```python
from build123d import *

# Parameters (mm, degrees)
SKETCH2_W           = 30
SKETCH2_H           = 10
BOSS_EXTRUDE1_DEPTH = 6.35
SKETCH3_W           = 35.56
SKETCH3_H           = 10
CUT_EXTRUDE1_DEPTH  = 6.35


with BuildPart() as part:
    # Sketch2 → Boss-Extrude1 (new body)
    with BuildSketch(Plane.XY):
        Polygon((12.244662888, 165.1), (24.944662888, 165.1), (24.944662888, 158.75), (35.263412888, 158.75), (35.263412888, 150.8125), (32.882162888, 150.8125), (32.882162888, 147.6375), (35.263412888, 147.6375), (35.263412888, 144.4625), (40.025912888, 144.4625), (40.025912888, 147.6375), (42.407162888, 147.6375), (42.407162888, 150.8125), (40.025912888, 150.8125), (40.025912888, 158.75), (50.344662888, 158.75), (50.344662888, 165.1), (63.044662888, 165.1), (63.044662888, 158.75), (75.744662888, 158.75), (75.744662888, 6.35), (63.044662888, 6.35), (63.044662888, 0), (50.344662888, 0), (50.344662888, 6.35), (40.025912888, 6.35), (40.025912888, 14.2875), (42.407162888, 14.2875), (42.407162888, 17.4625), (40.025912888, 17.4625), (40.025912888, 20.6375), (35.263412888, 20.6375), (35.263412888, 17.4625), (32.882162888, 17.4625), (32.882162888, 14.2875), (35.263412888, 14.2875), (35.263412888, 6.35), (24.944662888, 6.35), (24.944662888, 0), (12.244662888, 0), (12.244662888, 6.35), (-0.455337112, 6.35), (-0.455337112, 158.75), (12.244662888, 158.75), align=None)
        with Locations((37.644662886, 55.8)):
            Rectangle(SKETCH2_W, SKETCH2_H, mode=Mode.SUBTRACT)
    extrude(amount=BOSS_EXTRUDE1_DEPTH)

    # Sketch3 → Cut-Extrude1 (cut)
    with BuildSketch(Plane.XY.offset(6.35)):
        with Locations((37.623375509, 55.8)):
            Rectangle(SKETCH3_W, SKETCH3_H)
    extrude(amount=-CUT_EXTRUDE1_DEPTH, mode=Mode.SUBTRACT)


solid = part.part
```
Read the model definition and answer for the solid it produces. Units are mm, in the model's axes. A direction names the side the tool comes from. Give positions to 0.01 mm unless a question says otherwise; leave off trailing zeros. Loops run counter-clockwise (first coordinate to the right, second up) from the corner with the lowest first, then second, coordinate; pieces in that order, holes last.
Item 1: The mould has two halves that part along Y. Classify faces 5 (the flat face through (19, 0, 3)), 6 (the flat face through (45, 158.75, 3)), 7 (the flat face through (37, 60.8, 3)): released by +Y, released by -Y, zero draft, split by the parting line, or undercut.
Item 2: Find the intervals of material crossed by line 1 along X through (y, z) = (153, 5.25); line 2 along X through (y, z) = (59, 6); line 3 along Y through (x, z) = (38, 0.5), in increasing order.
Item 3: The part is cut by section B-B (y = 146). Write down the section's boundary in (x, z), and give its area (3 significant figures).
Item 4: Each of these flat-tipped pins is pushed along its axis until it touches: pin 1 Ø1.9 at (x, z) = (47.5, 2.5) entering from -Y; pin 2 Ø2 at (x, z) = (47.5, 4) entering from +Y; pin 3 Ø3 at (y, z) = (161, 3.5) entering from +X. Where does it stop, or does it pass through?
Item 5: For faces 1 (the flat face through (35.263, 146, 3)), 2 (the flat face through (42.407, 16, 3)), 3 (the flat face through (69, 6.35, 3)), 4 (the flat face through (35.263, 19, 3)), determine the directions among +Z, -Z, +X, -X, +Y, -Y from which every point of the face is accessible in a straight line to the end or side of a thin tool.
Item 6: The part is cut by section C-C (x = 6.5). Write down the section's boundary in (y, z), and give its area (3 significant figures).
Item 7: The part is cut by section A-A (x = 52). Write down the section's boundary in (y, z), and give its area (3 significant figures).
Taken from the geometry:
1. face 5: released by -Y
1. face 6: released by +Y
1. face 7: undercut
2. line 1: x = -0.46 to 35.26, 40.03 to 75.74
2. line 2: x = -0.46 to 19.84, 55.4 to 75.74
2. line 3: y = 20.64 to 50.8, 60.8 to 144.46
3. outline: (-0.46, 0) - (35.26, 0) - (35.26, 6.35) - (-0.46, 6.35) - close; (40.03, 0) - (75.74, 0) - (75.74, 6.35) - (40.03, 6.35) - close
3. area: 454 mm2
4. pin 1: stops at y = 6.35
4. pin 2: stops at y = 158.75
4. pin 3: stops at x = 63.04
5. face 1: +Z, -Z, +Y
5. face 2: +Z, -Z
5. face 3: +Z, -Z, +X, -Y
5. face 4: +Z, -Z, -Y
6. outline: (6.35, 0) - (158.75, 0) - (158.75, 6.35) - (6.35, 6.35) - close
6. area: 968 mm2
7. outline: (0, 0) - (50.8, 0) - (50.8, 6.35) - (0, 6.35) - close; (60.8, 0) - (165.1, 0) - (165.1, 6.35) - (60.8, 6.35) - close
7. area: 985 mm2
